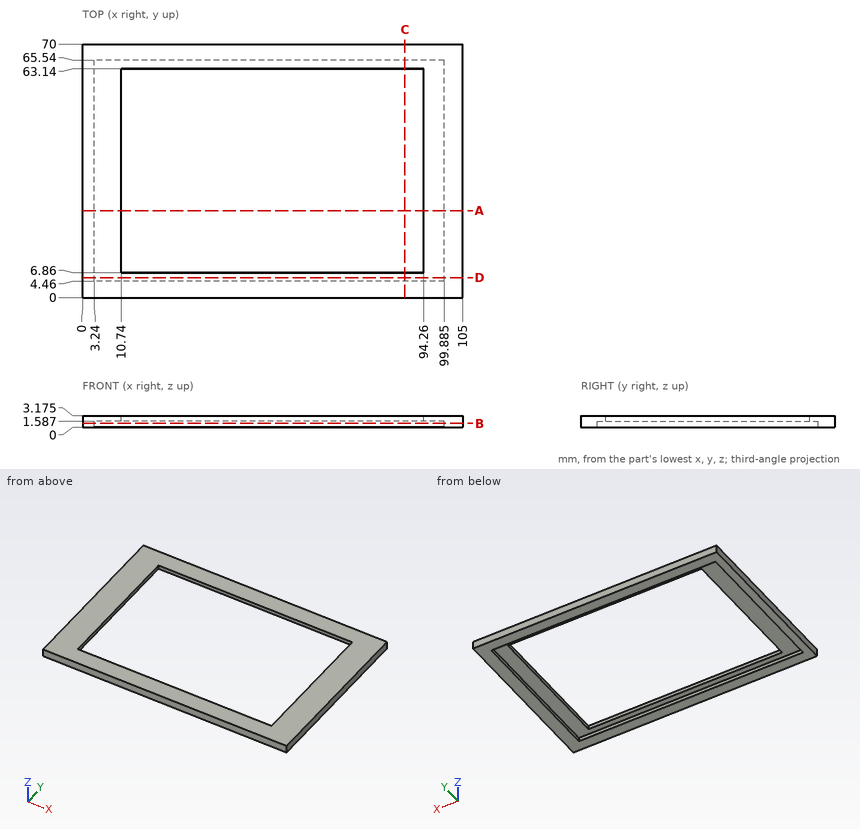
Here's the drawing with two shaded views (mm, measured from the low corner). I have some questions. Round coordinates to 2 decimals unless told otherwise and drop trailing zeros. Write each loop counter-clockwise with the first axis right and the second up, starting at its lowest first coordinate (ties: lowest second). Pieces come first, ordered by that corner, then holes.
(1) Suppose I cut it at C-C on x = 89. Write out the boundary of the cut face in (y, z) (1 decimal).
Findings below:
outline: (0, 0) - (4.5, 0) - (4.5, 1.6) - (6.9, 1.6) - (6.9, 3.2) - (0, 3.2) - close; (63.1, 1.6) - (65.5, 1.6) - (65.5, 0) - (70, 0) - (70, 3.2) - (63.1, 3.2) - close
(2) Suppose I cut it at D-D on y = 5.5. Write out the boundary of the cut face in (x, z) (1 decimal), and give its area (3 significant figures).
Findings below:
outline: (0, 0) - (3.2, 0) - (3.2, 1.6) - (99.9, 1.6) - (99.9, 0) - (105, 0) - (105, 3.2) - (0, 3.2) - close
area: 180 mm2
(3) Suppose I cut it at A-A on y = 24. Write out the boundary of the cut face in (x, z) (1 decimal).
Findings below:
outline: (0, 0) - (3.2, 0) - (3.2, 1.6) - (10.7, 1.6) - (10.7, 3.2) - (0, 3.2) - close; (94.3, 1.6) - (99.9, 1.6) - (99.9, 0) - (105, 0) - (105, 3.2) - (94.3, 3.2) - close
(4) Suppose I cut it at B-B on z = 1. Write out the boundary of the cut face in (x, y) (1 decimal), and give its area (3 significant figures).
Findings below:
outline: (0, 0) - (105, 0) - (105, 70) - (0, 70) - close; hole (3.2, 4.5) - (99.9, 4.5) - (99.9, 65.5) - (3.2, 65.5) - close
area: 1,450 mm2
(5) For pin 1 (0.8 mm diameter, centred on y = 38, z = 1, fed in from -X), with a flat end and sliding along its axis, tell me the tip position at first contact or that it passes through.
Findings below:
pin 1: stops at x = 0
(6) If I drill on probe 1 along Y at (x, z) = (30, 2.4); probe 2 along Y at (x, z) = (25, 1.4); probe 3 along X at (y, z) = (49.5, 1.5) (1 decimal), over which ranges is the centre line in solid material (lowest first)?
Findings below:
probe 1: y = 0 to 6.86, 63.14 to 70
probe 2: y = 0 to 4.46, 65.54 to 70
probe 3: x = 0 to 3.2, 99.9 to 105
